Geometry: final body of the model. Coordinates: model frame, mm. Give positions to 0.01 mm unless a question says otherwise; leave off trailing zeros. Order: outer loops, then holes, each group sorted by start corner. A loop starts at its lowest first (then second) coordinate and runs counter-clockwise, first axis right, second up. Notation, with made-up numbers: (21.25, 84) -> (31.25, 84) arc R17 cw to (31.25, 102) -> close; hole circle Ø1 at (66.5, -29). An arc over 180 degrees is marked (long way). Answer in a Markdown table with one row per item. Add a question column.
Q1. Cut plane D-D on x = -3.25. Return the cut outline in (y, z), and give its area (3 significant figures).
Q2. Line query: line 1 along Y through (x, z) = (0, 0.5); line 2 along Y through (x, z) = (-1, 0.2); line 3 along Y through (x, z) = (3.5, 1.1). Output: solid intervals per line, ascending. Write a range as from..to.
Q3. Cut plane C-C on z = 0.3. Count the separate pieces of the cut face and the enclosed holes in it, and give its area (3 significant figures).
Q4. Cut plane A-A on x = 0. Return the cut outline in (y, z).
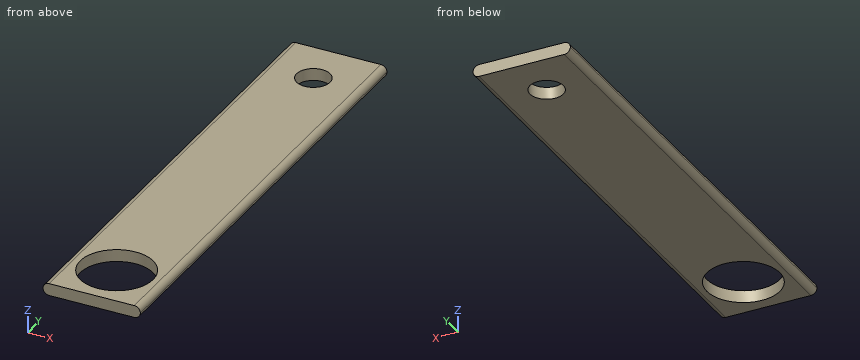
Autodesk Inventor part; units mm, degrees
ref_plane "YZ Plane" through (0, 0, 0) normal (1, 0, 0) x (0, 1, 0)
ref_plane "XZ Plane" through (0, 0, 0) normal (0, 1, 0) x (-1, 0, 0)
ref_plane "XY Plane" through (0, 0, 0) normal (0, 0, 1) x (1, 0, 0)
sketch "Sketch1" plane through (0, 0, 0) normal (0, 0, 1) x (1, 0, 0)
  circle A0 centre (0, 25) radius 2.1828
  circle A1 centre (0, -25) radius 4.7625
  line L0 (-6.35, -31.35) -> (6.35, -31.35)
  line L1 (6.35, -31.35) -> (6.35, 31.35)
  line L2 (6.35, 31.35) -> (-6.35, 31.35)
  line L3 (-6.35, 31.35) -> (-6.35, -31.35)
  line L4 (-6.35, -31.35) -> (6.35, 31.35) construction
  line L5 (6.35, -31.35) -> (-6.35, 31.35) construction
  point P0 (0, 0)
  dimension "d0" = 4.3656
  dimension "d1" = 9.525
  dimension "d2" = 25
  dimension "d3" = 50
  dimension "d4" = 12.7
  dimension "d5" = 6.35
extrude "Extrusion1" add sketch "Sketch1" along normal blind 1.5875
fillet "Fillet1" radius 0.7937 4 edges at (-6.35, 0, 0) (-6.35, 0, 1.5875) (6.35, 0, 0) (6.35, 0, 1.5875)
properties part number "Part J"
Completed:
| question | item | result |
|---|---|---|
| 1 | outline | (-31.35, 0) -> (-28.48, 0) -> (-28.48, 1.59) -> (-31.35, 1.59) -> close; (-21.52, 0) -> (31.35, 0) -> (31.35, 1.59) -> (-21.52, 1.59) -> close |
| 1 | area | 88.5 mm² |
| 2 | line 1 | y = -31.35..-29.76, -20.24..22.82, 27.18..31.35 |
| 2 | line 2 | y = -31.35..-29.66, -20.34..23.06, 26.94..31.35 |
| 2 | line 3 | y = -31.35..-28.23, -21.77..31.35 |
| 3 | separate pieces | 1 |
| 3 | enclosed holes | 2 |
| 3 | area | 688 mm² |
| 4 | outline | (-31.35, 0) -> (-29.76, 0) -> (-29.76, 1.59) -> (-31.35, 1.59) -> close; (-20.24, 0) -> (22.82, 0) -> (22.82, 1.59) -> (-20.24, 1.59) -> close; (27.18, 0) -> (31.35, 0) -> (31.35, 1.59) -> (27.18, 1.59) -> close |
